Input: part model. Units: mm. Frame: model coordinates. Face numbers are marked on the shaded views. A direction names the side the tool comes from. Round coordinates to 2 decimals unless told otherwise and drop trailing zeros. Loops run counter-clockwise (first coordinate to the right, second up) from the corner with the lowest first, then second, coordinate; pieces in that order, holes last. Notation, with made-up numbers: (-38, -0.5) - (-26, -0.5) arc R29 ccw to (-26, 36.5) - close; hole circle Ø10 at (66, -10). An arc over 180 degrees is marked (long way). Use CSV: the item, a comma, the result in double quotes. Start each with the question number.
1. Material intervals for probe 1 along X at (y, z) = (-0.5, 38.5); probe 2 along Z at (x, y) = (-6.25, 6.5); probe 3 along X at (y, z) = (-0.25, 6), sorted ascending. Write a range as from..to.
2. Pin query (flat end, axial travel): P1, Ø2, axis at x = 2.5, y = -7, coming from the -Z side; P2, Ø5, axis at y = 1.5, z = 37, coming from the +X side; P3, Ø1, axis at y = 3, z = 24.5, coming from the -X side; P4, Ø6, axis at x = -2.5, z = 19.5, coming from the +Y side. Return the tip coordinate at first contact, or that it passes through.
3. Access query for the marked faces 1, 2 and 3. Directions: +Z, -Z, +X, -X, +Y, -Y. A direction counts if a zero-diameter tool reaches every point of the face in a straight line with its end or side. Return the directions, or none.
4. Cut plane C-C (x = 8.5). Return loops of the section in (y, z).
5. Cut plane D-D (y = -3). Return loops of the section in (x, z).
6. Cut plane A-A (y = 0). Return loops of the section in (x, z), and give its area (3 significant figures).
7. Cut plane B-B (z = 6). Return loops of the section in (x, y), and give its area (3 significant figures).
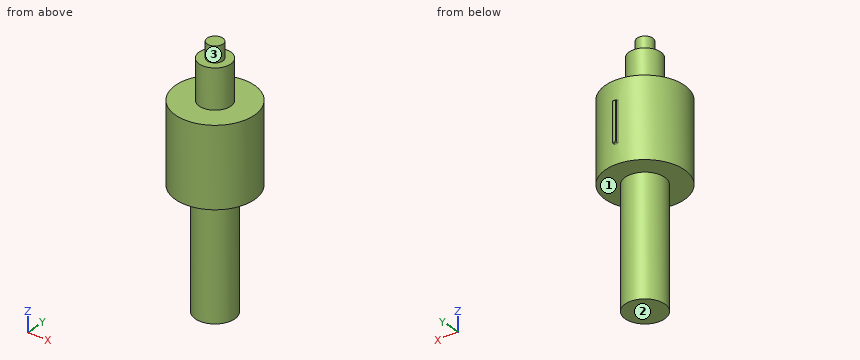
```python
from build123d import *

# Parameters (mm, degrees)
SKETCH1_R           = 5
BOSS_EXTRUDE1_DEPTH = 30
SKETCH2_R           = 10
BOSS_EXTRUDE2_DEPTH = 20
SKETCH3_R           = 4
BOSS_EXTRUDE3_DEPTH = 10
SKETCH4_R           = 2
BOSS_EXTRUDE4_DEPTH = 4
BOSS_EXTRUDE5_START = -5
BOSS_EXTRUDE5_DEPTH = 10
FILLET1_R           = 0.2


with BuildPart() as part:
    # Sketch1 → Boss-Extrude1 (new body)
    with BuildSketch(Plane.XY):
        Circle(SKETCH1_R)
    extrude(amount=BOSS_EXTRUDE1_DEPTH)

    # Sketch2 → Boss-Extrude2 (add)
    with BuildSketch(Plane.XY.offset(30)):
        Circle(SKETCH2_R)
    extrude(amount=BOSS_EXTRUDE2_DEPTH)

    # Sketch3 → Boss-Extrude3 (add)
    with BuildSketch(Plane.XY.offset(50)):
        Circle(SKETCH3_R)
    extrude(amount=BOSS_EXTRUDE3_DEPTH)

    # Sketch4 → Boss-Extrude4 (add)
    with BuildSketch(Plane.XY.offset(60)):
        Circle(SKETCH4_R)
    extrude(amount=BOSS_EXTRUDE4_DEPTH)

    # Sketch5 → Boss-Extrude5 (add)
    with BuildSketch(Plane(origin=(0, 0, 30), x_dir=(-1, 0, 0), z_dir=(0, 0, -1)).offset(BOSS_EXTRUDE5_START)):
        with BuildLine():
            Line((-0.464729596, 10.560180083), (0.535270404, 10.560180083))
            Line((0.535270404, 10.560180083), (0.535270404, 9.960180083))
            ThreePointArc((0.535270404, 9.960180083), (0.035314802, 9.97449019), (-0.464729596, 9.963720595))
            Line((-0.464729596, 9.963720595), (-0.464729596, 10.560180083))
        make_face()
    extrude(amount=-BOSS_EXTRUDE5_DEPTH)

    # Fillet1
    fillet1_edges = [part.edges().sort_by_distance(p)[0] for p in [
        (-0.035314575, 9.999937644, 35),
        (-0.535270404, 9.985664004, 40),
        (0.464729596, 9.989195483, 40),
        (-0.035314575, 9.999937644, 45),
        (0.464729596, 10.274687783, 45),
        (-0.535270404, 10.272922043, 45),
        (-0.535270404, 10.560180083, 40),
        (-0.035270404, 10.560180083, 45),
        (0.464729596, 10.560180083, 40),
        (-0.535270404, 10.272922043, 35),
        (-0.035270404, 10.560180083, 35),
        (0.464729596, 10.274687783, 35),
    ]]
    fillet(fillet1_edges, radius=FILLET1_R)


solid = part.part
```
Established:
1,probe 1,"x = -9.99..9.99"
1,probe 2,"z = 30..50"
1,probe 3,"x = -4.99..4.99"
2,P1,"stops at z = 30"
2,P2,"stops at x = 10"
2,P3,"stops at x = -4.33"
2,P4,"stops at y = 5"
3,face 1,"-Z"
3,face 2,"-Z, +X, -X, +Y, -Y"
3,face 3,"+Z"
4,outline,"(-5.27, 30) - (5.27, 30) - (5.27, 50) - (-5.27, 50) - close"
5,outline,"(-9.54, 30) - (-4, 30) - (-4, 0) - (4, 0) - (4, 30) - (9.54, 30) - (9.54, 50) - (2.65, 50) - (2.65, 60) - (-2.65, 60) - (-2.65, 50) - (-9.54, 50) - close"
6,outline,"(-10, 30) - (-5, 30) - (-5, 0) - (5, 0) - (5, 30) - (10, 30) - (10, 50) - (4, 50) - (4, 60) - (2, 60) - (2, 64) - (-2, 64) - (-2, 60) - (-4, 60) - (-4, 50) - (-10, 50) - close"
6,area,"796 mm2"
7,outline,"circle Ø10 at (0, 0)"
7,area,"78.5 mm2"
